```python
from build123d import *

# Parameters (mm, degrees)
F0_W     = 152.4
F0_H     = 76.2
F1_DEPTH = 12.7
F2_R     = 3.81
F3_DEPTH = 25.4
F4_R     = 3.81
F4_R_2   = 3.716512
F5_DEPTH = 12.701


with BuildPart() as f1:
    # F0 (on Top) → F1 (new body)
    with BuildSketch(Plane.XY):
        with Locations((16.127278, 8.251033)):
            Rectangle(F0_W, F0_H)
    extrude(amount=F1_DEPTH)

    # F2 (on face) → F3 (cut)
    with BuildSketch(Plane.XY.offset(12.7)):
        Circle(F2_R)
    extrude(amount=-F3_DEPTH, mode=Mode.SUBTRACT)

    # F4 (on face) → F5 (cut, through all)
    with BuildSketch(Plane.XY.offset(12.7)):
        with Locations((18.605455, 0)):
            Circle(F4_R)
        with Locations((41.206335, 0)):
            Circle(F4_R_2)
    extrude(amount=-F5_DEPTH, mode=Mode.SUBTRACT)


solid = f1.part
```
Geometry: final body of the model. Coordinates: model frame, mm. Round coordinates to 2 decimals unless told otherwise and drop trailing zeros. Order: outer loops, then holes, each group sorted by start corner. A loop starts at its lowest first (then second) coordinate and runs counter-clockwise, first axis right, second up. Notation, with made-up numbers: M 74,-16.5 L 126,-16.5 A27 cw 126,5.5 Z; hole C 15,-40 d11. An arc over 180 degrees is marked long. One line per item, written item: value.
(1) Pull-direction query (Y, two-part tool) for faces 1 (the flat face through (15, -29.849, 6)), 2 (the flat face through (15, 9, 0)), 3 (the cylindrical face through (14.8, 0.2, 6.4)), 4 (the flat face through (15, 46.351, 6)); classes: pulls with the +Y half, pulls with the -Y half, needs draft (parallel to the pull), parting line crosses it, or undercut.
Result sheet:
face 1: pulls with the -Y half
face 2: needs draft
face 3: undercut
face 4: pulls with the +Y half
(2) Cut plane B-B (y = 0). Return the cut outline in (x, z), and give its area (3 significant figures).
Result sheet:
outline: M -60.07,0 L -3.81,0 L -3.81,12.7 L -60.07,12.7 Z; M 3.81,0 L 14.8,0 L 14.8,12.7 L 3.81,12.7 Z; M 22.42,0 L 37.49,0 L 37.49,12.7 L 22.42,12.7 Z; M 44.92,0 L 92.33,0 L 92.33,12.7 L 44.92,12.7 Z
area: 1,650 mm2
(3) Line query: probe 1 along Y at (x, z) = (0, 6.5); probe 2 along X at (y, z) = (-3, 1); probe 3 along Y at (x, z) = (43, 6.5). Output: solid intervals per line, ascending. Write a range as [from, to].
Result sheet:
probe 1: [-29.85, -3.81], [3.81, 46.35]
probe 2: [-60.07, -2.35], [2.35, 16.26], [20.95, 39.01], [43.4, 92.33]
probe 3: [-29.85, -3.26], [3.26, 46.35]
(4) Cut plane A-A (x = 0). Return the cut outline in (y, z), and give its area (3 significant figures).
Result sheet:
outline: M -29.85,0 L -3.81,0 L -3.81,12.7 L -29.85,12.7 Z; M 3.81,0 L 46.35,0 L 46.35,12.7 L 3.81,12.7 Z
area: 871 mm2
